```python
from build123d import *

# Parameters (mm, degrees)
SKETCH1_R           = 7.5
BOSS_EXTRUDE1_DEPTH = 5
SKETCH2_R           = 1.3
CUT_EXTRUDE1_DEPTH  = 3
FILLET1_R           = 2
SKETCH3_R           = 2.5
BOSS_EXTRUDE2_DEPTH = 20


with BuildPart() as part:
    # Sketch1 → Boss-Extrude1 (new body)
    with BuildSketch(Plane(origin=(0, 0, 0), x_dir=(1, 0, 0), z_dir=(0, 1, 0))):
        with Locations(Location((0, 0, 0), (0, 0, 270))):
            Circle(SKETCH1_R)
    extrude(amount=BOSS_EXTRUDE1_DEPTH)

    # Sketch2 → Cut-Extrude1 (cut)
    with BuildSketch(Plane(origin=(0, 5, 0), x_dir=(1, 0, 0), z_dir=(0, 1, 0))):
        with Locations(Location((0, 5, 0), (0, 0, 270))):
            Circle(SKETCH2_R)
        with Locations(Location((5, 0, 0), (0, 0, 270))):
            Circle(SKETCH2_R)
        with Locations(Location((0, -5, 0), (0, 0, 270))):
            Circle(SKETCH2_R)
        with Locations(Location((-5, 0, 0), (0, 0, 270))):
            Circle(SKETCH2_R)
    extrude(amount=-CUT_EXTRUDE1_DEPTH, mode=Mode.SUBTRACT)

    # Fillet1
    fillet1_edges = [part.edges().sort_by_distance(p)[0] for p in [
        (0, 0, -7.5),
    ]]
    fillet(fillet1_edges, radius=FILLET1_R)

    # Sketch3 → Boss-Extrude2 (add)
    with BuildSketch(Plane.XZ):
        with Locations(Location((0, 0, 0), (0, 0, 90))):
            Circle(SKETCH3_R)
    extrude(amount=BOSS_EXTRUDE2_DEPTH)


solid = part.part
```
Design review of the part built by this model. Coordinates are the model's own, in mm. A direction names the side the tool comes from. Coordinates: 2 decimals unless noted, no trailing zeros. Order: outer loops, then holes, each group sorted by start corner. A loop starts at its lowest first (then second) coordinate and runs counter-clockwise, first axis right, second up.
1) Take a section at D-D, the plane y = 0.75. Give the boundary of the cut face in (x, z).
2) Take a section at B-B, the plane x = 0. Give the boundary of the cut face in (y, z), and give its area (3 significant figures).
3) Clearance check with flat-ended pins moving along their axes: pin 1 (3 mm diameter, centred on x = -5, z = 0.5, fed in from +Y); pin 2 (0.8 mm diameter, centred on x = 4.5, z = 0.5, fed in from +Y); pin 3 (2.5 mm diameter, centred on x = 5, z = 0, fed in from -Y); pin 4 (6 mm diameter, centred on x = 2.5, y = -9.5, fed in from +Z). State where each tip first meets the part, or that it passes through.
4) For faces 4 (the flat face through (0, 0, -3)), 5 (the flat face through (0, -20, 0)), 6 (the cylindrical face through (0.39, 3.52, -3.76)), list the 3-axis set-ups (+Z, -Z, +X, -X, +Y, -Y) from which the entire face can be reached by the end or side of a thin tool; tool diameter is ignored.
5) Mouldability with a two-part tool opening along X and no side actions: class faces 1 (the flat face through (0, 5, 0)), 2 (the flat face through (0, 2, -5)), 3 (the cylindrical face through (2.44, -9.86, -0.54)) as +X half, -X half, draft (parallel to the pull), parting line (faces both ways), or undercut.
6) Take a section at C-C, the plane y = -17.5. Give the boundary of the cut face in (x, z).
7) Take a section at A-A, the plane z = 0. Give the boundary of the cut face in (x, y).
8) Wall thickness on line 1 along X through (y, z) = (4.35, 0); line 2 along Y through (x, z) = (1.5, -5.25); line 3 along Y through (x, z) = (-0.75, 5): over which ranges is each line inside the solid? List them lowest first.
Returned:
1. outline: circle Ø14.12 at (0, 0)
2. outline: (-20, -2.5) - (0, -2.5) - (0, -5.5) arc R2 ccw to (2, -7.5) - (5, -7.5) - (5, -6.3) - (2, -6.3) - (2, -3.7) - (5, -3.7) - (5, 3.7) - (2, 3.7) - (2, 6.3) - (5, 6.3) - (5, 7.5) - (2, 7.5) arc R2 ccw to (0, 5.5) - (0, 2.5) - (-20, 2.5) - close
2. area: 158 mm2
3. pin 1: stops at y = 5
3. pin 2: stops at y = 2
3. pin 3: stops at y = 0
3. pin 4: stops at z = 2.5
4. face 4: -Y
4. face 5: +Z, -Z, +X, -X, -Y
4. face 6: +Y
5. face 1: draft
5. face 2: undercut
5. face 3: parting line
6. outline: circle Ø5 at (0, 0)
7. outline: (-7.5, 2) arc R2 ccw to (-5.5, 0) - (-2.5, 0) - (-2.5, -20) - (2.5, -20) - (2.5, 0) - (5.5, 0) arc R2 ccw to (7.5, 2) - (7.5, 5) - (6.3, 5) - (6.3, 2) - (3.7, 2) - (3.7, 5) - (-3.7, 5) - (-3.7, 2) - (-6.3, 2) - (-6.3, 5) - (-7.5, 5) - close
8. line 1: x = -7.5 to -6.3, -3.7 to 3.7, 6.3 to 7.5
8. line 2: y = 0 to 5
8. line 3: y = 0 to 2
